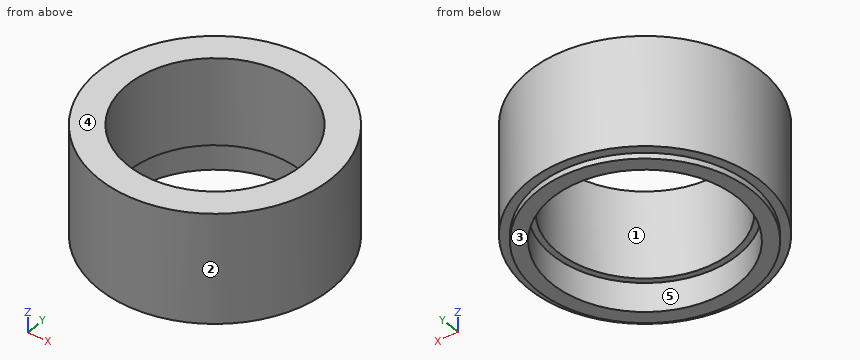
from build123d import *

# Parameters (mm, degrees)
SKETCH_1_R          = 20
EXTRUDE_1_DEPTH     = 20
SKETCH_4_R          = 20
SKETCH_4_R_2        = 18.5
CUT_EXTRUDE_3_DEPTH = 1
SKETCH_3_R          = 16
CUT_EXTRUDE_2_DEPTH = 5
SKETCH_6_R          = 15
CUT_EXTRUDE_4_DEPTH = 21


with BuildPart() as part:
    # ｽｹｯﾁ1 → ﾎﾞｽ - 押し出し1 (new body)
    with BuildSketch(Plane.XY):
        Circle(SKETCH_1_R)
    extrude(amount=EXTRUDE_1_DEPTH)

    # ｽｹｯﾁ4 → ｶｯﾄ - 押し出し3 (cut)
    with BuildSketch(Plane(origin=(0, 0, 0), x_dir=(-1, 0, 0), z_dir=(0, 0, -1))):
        Circle(SKETCH_4_R)
        Circle(SKETCH_4_R_2, mode=Mode.SUBTRACT)
    extrude(amount=-CUT_EXTRUDE_3_DEPTH, mode=Mode.SUBTRACT)

    # ｽｹｯﾁ3 → ｶｯﾄ - 押し出し2 (cut)
    with BuildSketch(Plane(origin=(0, 0, 0), x_dir=(-1, 0, 0), z_dir=(0, 0, -1))):
        Circle(SKETCH_3_R)
    extrude(amount=-CUT_EXTRUDE_2_DEPTH, mode=Mode.SUBTRACT)

    # ｽｹｯﾁ6 → ｶｯﾄ - 押し出し4 (cut, through all)
    with BuildSketch(Plane.XY.offset(20)):
        Circle(SKETCH_6_R)
    extrude(amount=-CUT_EXTRUDE_4_DEPTH, mode=Mode.SUBTRACT)


solid = part.part
The listing builds one solid part. Answer for the finished solid, in the listing's coordinates (mm). Face numbers are marked on the shaded views. A direction names the side the tool comes from. Give positions to 0.01 mm unless a question says otherwise; leave off trailing zeros. Order: outer loops, then holes, each group sorted by start corner. A loop starts at its lowest first (then second) coordinate and runs counter-clockwise, first axis right, second up. Notation, with made-up numbers: (20.5, 30.25) - (45.5, 30.25) arc R26 cw to (45.5, 62.25) - close; hole circle Ø10 at (32.5, -20). An arc over 180 degrees is marked (long way). One line per item, written item: value. Start each with the question number.
1) The mould has two halves that part along X. Classify the marked faces 1, 2 and 3: released by +X, released by -X, zero draft, split by the parting line, or undercut.
2) A cutting plane is placed at C-C on z = 8.75. Give the vertices of the cut face in (x, y).
3) A tool of negligible diameter and unlimited length cuts with its end or side. For the marked faces 4 and 5, from which of +Z, -Z, +X, -X, +Y, -Y can it reach the whole face along a straight path? Write none if from no direction.
4) A cutting plane is placed at A-A on y = 0. Give the vertices of the cut face in (x, z), then the cut area to 3 significant figures.
5) Given pin 1 Ø6 at (x, z) = (-14.5, 10.5) entering from +Y; pin 2 Ø4 at (x, z) = (-11.5, 14) entering from -Y; pin 3 Ø8 at (y, z) = (12.5, 14) entering from +X, each flat-ended and moving along its own axis, determine where each tip first touches the part or whether it passes through.
6) Find the intervals of material crossed by L1, parallel to Y at x = 0, z = 2.6; L2, parallel to Y at x = 0, z = 16; L3, parallel to Z at x = 15.5, y = 3.5, in increasing order.
Answer sheet:
1. face 1: undercut
1. face 2: split by the parting line
1. face 3: zero draft
2. outline: circle Ø40 at (0, 0); hole circle Ø30 at (0, 0)
3. face 4: +Z, +X, -X, +Y, -Y
3. face 5: -Z
4. outline: (-20, 1) - (-18.5, 1) - (-18.5, 0) - (-16, 0) - (-16, 5) - (-15, 5) - (-15, 20) - (-20, 20) - close; (15, 5) - (16, 5) - (16, 0) - (18.5, 0) - (18.5, 1) - (20, 1) - (20, 20) - (15, 20) - close
4. area: 187 mm2
5. pin 1: stops at y = 16.36
5. pin 2: stops at y = -17.6
5. pin 3: stops at x = 18.1
6. L1: y = -20 to -16, 16 to 20
6. L2: y = -20 to -15, 15 to 20
6. L3: z = 5 to 20
